```python
from build123d import *

# Parameters (mm, degrees)
F0_W     = 40
F0_H     = 40
F1_DEPTH = 5.842


with BuildPart() as f1:
    # F0 (on Top) → F1 (new body)
    with BuildSketch(Plane.XY):
        Polygon((-20, 25), (-25, 25), (-30.842, 25), (-30.842, 20), (-25, 20), (-25, 6.666667), (-30.842, 6.666667), (-30.842, -6.666667), (-25, -6.666667), (-25, -20), (-30.842, -20), (-30.842, -25), (-25, -25), (-20, -25), (-20, -30.842), (-6.666667, -30.842), (-6.666667, -25), (6.666667, -25), (6.666667, -30.842), (20, -30.842), (20, -25), (25, -25), (30.842, -25), (30.842, -20), (25, -20), (25, -6.666667), (30.842, -6.666667), (30.842, 6.666667), (25, 6.666667), (25, 20), (30.842, 20), (30.842, 25), (25, 25), (20, 25), (20, 30.842), (6.666667, 30.842), (6.666667, 25), (-6.666667, 25), (-6.666667, 30.842), (-20, 30.842), align=None)
        with Locations((0.947482, -0.06855)):
            Rectangle(F0_W, F0_H, mode=Mode.SUBTRACT)
    extrude(amount=F1_DEPTH)


solid = f1.part
```
For this review, take the finished solid that the model builds, in its own axes (mm). A direction names the side the tool comes from. Round coordinates to 2 decimals unless told otherwise and drop trailing zeros. Write each loop counter-clockwise with the first axis right and the second up, starting at its lowest first coordinate (ties: lowest second). Pieces come first, ordered by that corner, then holes. Notation, with made-up numbers: (37.5, -31.75) -> (70.5, -31.75) arc R12 ccw to (70.5, -27.75) -> close; hole circle Ø8 at (40, 7). An arc over 180 degrees is marked (long way). One line per question, with ' | ' between items. Start each with the question number.
(1) Mouldability with a two-part tool opening along Y and no side actions: class faces 6 (the face through (0, -25, 3)), 7 (the face through (-25, 13, 3)), 8 (the face through (-6.667, 28, 3)) as released by +Y, released by -Y, zero draft, split by the parting line, or undercut.
(2) Add section B-B, the plane x = -3.5. Write out the cut boundary in (y, z), plus the area to 3 significant figures.
(3) Add section A-A, the plane y = 10.5. Write out the cut boundary in (x, z), plus the area to 3 significant figures.
(4) Tool access review of faces 1 (the face through (-20, 28, 3)), 2 (the face through (-6.667, -28, 3)), 3 (the face through (-28, -6.667, 3)), 4 (the face through (28, 6.667, 3)), 5 (the face through (-25, -25, 3)): name each direction out of +Z, -Z, +X, -X, +Y, -Y from which nothing blocks a thin tool from reaching the whole face with its end or side.
(5) Add section C-C, the plane x = 22. Write out the cut boundary in (y, z).
(6) Insertion check: P1, Ø1, axis at y = 10, z = 1, coming from the -X side; P2, Ø1.8, axis at y = -28, z = 4, coming from the -X side; P3, Ø1.8, axis at x = -27, z = 1.5, coming from the +Y side. Each pin has a flat end and moves straight along its axis. Give the tip position at first contact, or say it passes through.
(7) For line 1 along Y through (x, z) = (27, 4.3); line 2 along X through (y, z) = (14.5, 0.8); line 3 along X through (y, z) = (1, 1.15), list the stretches that pass through material, from the lowest coordinate up. Write a range as from..to.
Answer list:
1) face 6: released by -Y | face 7: undercut | face 8: zero draft
2) outline: (-25, 0) -> (-20.07, 0) -> (-20.07, 5.84) -> (-25, 5.84) -> close; (19.93, 0) -> (25, 0) -> (25, 5.84) -> (19.93, 5.84) -> close | area: 58.4 mm²
3) outline: (-25, 0) -> (-19.05, 0) -> (-19.05, 5.84) -> (-25, 5.84) -> close; (20.95, 0) -> (25, 0) -> (25, 5.84) -> (20.95, 5.84) -> close | area: 58.4 mm²
4) face 1: +Z, -Z, -X, +Y | face 2: +Z, -Z, -Y | face 3: +Z, -Z, -X | face 4: +Z, -Z, +X | face 5: +Z, -Z, -X, -Y
5) outline: (-25, 0) -> (25, 0) -> (25, 5.84) -> (-25, 5.84) -> close
6) P1: x = -25 | P2: x = -20 | P3: y = 25
7) line 1: -25..-20, -6.67..6.67, 20..25 | line 2: -25..-19.05, 20.95..25 | line 3: -30.84..-19.05, 20.95..30.84
